CAD build for the part. Positions are in the model's coordinates, mm. A direction names the side the tool comes from. Give positions to 0.01 mm unless a question says otherwise; leave off trailing zeros. Loops run counter-clockwise (first coordinate to the right, second up) from the corner with the lowest first, then second, coordinate; pieces in that order, holes last. Notation, with made-up numbers: M 36.25,-23.75 L 63.25,-23.75 A19 cw 63.25,-4.75 Z; hole C 62.25,38.25 d3. An arc over 180 degrees is marked long. Answer as CSV lines item,"result".
Autodesk Inventor part; units mm, degrees
ref_plane "YZ Plane" through (0, 0, 0) normal (1, 0, 0) x (0, 1, 0)
ref_plane "XZ Plane" through (0, 0, 0) normal (0, 1, 0) x (-1, 0, 0)
ref_plane "XY Plane" through (0, 0, 0) normal (0, 0, 1) x (1, 0, 0)
sketch "Эскиз1" plane through (0, 0, 0) normal (0, 0, 1) x (1, 0, 0)
  point P0 (0, 0)
sketch "Эскиз2" plane through (0, 0, 0) normal (0, 1, 0) x (-1, 0, 0)
  line L0 (0, 15.5885) -> (13.5, 7.7942)
  line L1 (13.5, 7.7942) -> (13.5, -7.7942)
  line L2 (13.5, -7.7942) -> (0, -15.5885)
  line L3 (0, -15.5885) -> (-13.5, -7.7942)
  line L4 (-13.5, -7.7942) -> (-13.5, 7.7942)
  line L5 (-13.5, 7.7942) -> (0, 15.5885)
  point P0 (0, 0)
  point P1 (0, 0)
  dimension "d0" = 27
extrude "Выдавливание1" add sketch "Эскиз2" along normal blind 16
sketch "Эскиз3" plane through (0, 0, 0) normal (0, -1, 0) x (1, 0, 0)
  circle A0 centre (0, 0) radius 12.5
  dimension "d3" = 25
sketch "Эскиз4" plane through (0, 16, 0) normal (0, 1, 0) x (1, 0, 0)
  circle A0 centre (0, 0) radius 10.2935
  dimension "d4" = 20.587
extrude "Выдавливание2" cut sketch "Эскиз4" against normal blind 12
thread "Резьба1"
chamfer "Фаска1" distance 1.6 angle 45 1 edges at (-10.2935, 16, 0) measured on face at (10.1602, 8, 1.6512)
extrude "Выдавливание3" cut sketch "Эскиз3" against normal blind 1.154
properties part number "Поз10 Заглушка"
Q1. Pin check, flat tips, straight feed: P1, Ø12.5, axis at x = 0, z = 0, coming from the -Y side; P2, Ø4, axis at x = 2.5, y = 9, coming from the +Z side; P3, Ø3, axis at x = 10, y = 11, coming from the -Z side; P4, Ø6, axis at x = 5, z = 8.5, coming from the -Y side. Stop position of each tip, or through.
Solution:
P1,"stops at y = 1.15"
P2,"stops at z = 15.3"
P3,"stops at z = -10.68"
P4,"stops at y = 0"
Q2. Cut at C-C (y = 3). Write the cut outline in (x, z), and give its area (3 significant figures).
Solution:
outline,"M -13.5,-7.79 L 0,-15.59 L 13.5,-7.79 L 13.5,7.79 L 0,15.59 L -13.5,7.79 Z"
area,"631 mm²"
Q3. Mould opens along Z. For faces 4 (the flat face through (13.5, 8, 0)), 5 (the flat face through (0, 1.154, 0)), 6 (the flat face through (-6.655, 7.888, 11.746)) say: released by +Z, released by -Z, zero draft, split by the parting line, or undercut.
Solution:
face 4,"zero draft"
face 5,"undercut"
face 6,"released by +Z"
Q4. Cut at A-A (y = 13.5). Write the cut outline in (x, z), and give its area (3 significant figures).
Solution:
outline,"M -13.5,-7.79 L 0,-15.59 L 13.5,-7.79 L 13.5,7.79 L 0,15.59 L -13.5,7.79 Z; hole C 0,0 d20.59"
area,"298 mm²"
Q5. Wall check: line 1 (X direction, y = 8, z = 0); line 2 (Z direction, x = 0, y = 12.5); line 3 (Z direction, x = 0, y = 0.4). Give the ranges that are in metal, low to high. Write a range as [from, to].
Solution:
line 1,"x = [-13.5, -10.29], [10.29, 13.5]"
line 2,"z = [-15.59, -10.29], [10.29, 15.59]"
line 3,"z = [-15.59, -12.5], [12.5, 15.59]"
Q6. Which spindle directions (+Z, -Z, +X, -X, +Y, -Y) get a long thin tool onto all of the face, cutting with end or side? Do faces 1 (the cylindrical face through (-2.23, 9.27, 10.05)), 2 (the flat face through (6.655, 7.888, -11.746)), 3 (the cylindrical face through (11.923, 0.569, 3.755)). Say none if no direction does.
Solution:
face 1,"+Y"
face 2,"-Z, +X, +Y, -Y"
face 3,"-Y"
Q7. Cut at B-B (z = 0). Write the cut outline in (x, y), and give its area (3 significant figures).
Solution:
outline,"M -13.5,0 L -12.5,0 L -12.5,1.15 L 12.5,1.15 L 12.5,0 L 13.5,0 L 13.5,16 L 11.89,16 L 10.29,14.4 L 10.29,4 L -10.29,4 L -10.29,14.4 L -11.89,16 L -13.5,16 Z"
area,"154 mm²"
